Here's how the part is built. I have some questions about the finished solid (model axes, mm). Face numbers are marked on the shaded views. Give positions to 0.01 mm unless a question says otherwise; leave off trailing zeros. Loops run counter-clockwise (first coordinate to the right, second up) from the corner with the lowest first, then second, coordinate; pieces in that order, holes last.
Q1. I need wall thicknesses on probe 1 along Z at (x, y) = (0, 2.5); probe 2 along Y at (x, z) = (-8.5, 0); probe 3 along X at (y, z) = (3.5, 0). Which ranges of each line are inside material? Lowest first, please.
Q2. Thinking about a two-plate mould opening in Y: for the marked faces 1, 2 and 3, which applies, pulls with the +Y half, pulls with the -Y half, needs draft (parallel to the pull), parting line crosses it, or undercut?
Q3. I'm going to push flat-ended pins straight in: P1, Ø1.6, axis at x = 0, z = 0, coming from the -Y side; P2, Ø2, axis at y = 4, z = 0.5, coming from the -X side; P3, Ø3, axis at y = 3.5, z = 2, coming from the +X side. Where does each tip first touch, or does it pass through?
Q4. Suppose I cut it at D-D (x = -2.75). List the corners of the cut face in (y, z) for me, and give its area (3 significant figures).
Q5. Suppose I cut it at B-B (y = 1.5). List the corners of the cut face in (x, z) for me, and give its area (3 significant figures).
Q6. Suppose I cut it at A-A (z = 0). List the corners of the cut face in (x, y) for me.
Q7. Suppose I cut it at C-C (x = -0.25). List the corners of the cut face in (y, z) for me, and give its area (3 significant figures).
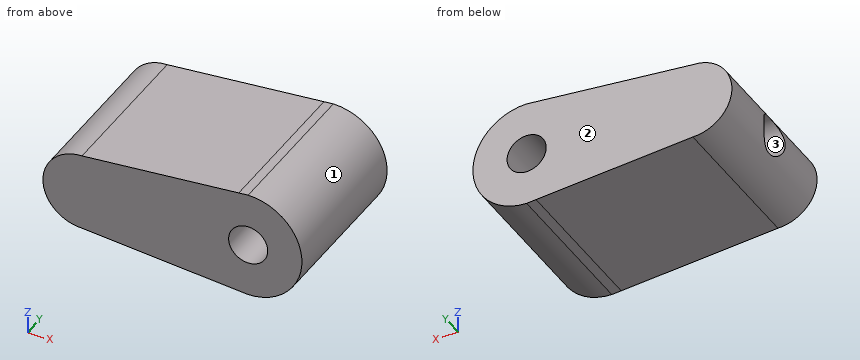
```python
from build123d import *

# Parameters (mm, degrees)
SKETCH1_R           = 1
BOSS_EXTRUDE1_DEPTH = 8
SKETCH2_R           = 1
CUT_EXTRUDE1_DEPTH  = 8


with BuildPart() as part:
    # Sketch1 → Boss-Extrude1 (new body)
    with BuildSketch(Plane(origin=(0, 0, 0), x_dir=(1, 0, 0), z_dir=(0, 1, 0))):
        with BuildLine():
            Line((-0.481545064, 2.70751073), (-8.5, 2))
            ThreePointArc((-8.5, 2), (-10.5, 0), (-8.5, -2))
            Line((-8.5, -2), (-0.481545064, -2.70751073))
            Line((-0.481545064, -2.70751073), (0, -2.75))
            ThreePointArc((0, -2.75), (2.75, 0), (0, 2.75))
            Line((0, 2.75), (-0.481545064, 2.70751073))
        make_face()
        Circle(SKETCH1_R, mode=Mode.SUBTRACT)
    extrude(amount=BOSS_EXTRUDE1_DEPTH)

    # Sketch2 → Cut-Extrude1 (cut)
    with BuildSketch(Plane.ZY.offset(10.5)):
        with Locations((0, 4)):
            Circle(SKETCH2_R)
    extrude(amount=-CUT_EXTRUDE1_DEPTH, mode=Mode.SUBTRACT)


solid = part.part
```
Solutions:
1. probe 1: z = -2.75 to -1, 1 to 2.75
1. probe 2: y = 0 to 3, 5 to 8
1. probe 3: x = -2.5 to -1, 1 to 2.75
2. face 1: needs draft
2. face 2: pulls with the +Y half
2. face 3: undercut
3. P1: passes through
3. P2: stops at x = -10.48
3. P3: stops at x = 2.7
4. outline: (0, -2.51) - (8, -2.51) - (8, 2.51) - (0, 2.51) - close; hole circle Ø2 at (4, 0)
4. area: 37.0 mm2
5. outline: (-8.5, -2) - (0, -2.75) arc R2.75 ccw to (0, 2.75) - (-8.5, 2) arc R2 ccw to start; hole circle Ø2 at (0, 0)
5. area: 55.4 mm2
6. outline: (-10.5, 0) - (-1, 0) - (-1, 8) - (-10.5, 8) - (-10.5, 5) - (-2.5, 5) - (-2.5, 3) - (-10.5, 3) - close; (1, 0) - (2.75, 0) - (2.75, 8) - (1, 8) - close
7. outline: (0, -2.73) - (8, -2.73) - (8, -0.97) - (0, -0.97) - close; (0, 0.97) - (8, 0.97) - (8, 2.73) - (0, 2.73) - close
7. area: 28.2 mm2
